Part model, mm, in its own coordinate system. A direction names the side the tool comes from. Coordinates: 2 decimals unless noted, no trailing zeros. Loops run counter-clockwise (first coordinate to the right, second up) from the corner with the lowest first, then second, coordinate; pieces in that order, holes last. Notation, with made-up numbers: M -31,-23.75 L 25,-23.75 A10 cw 25,-4.75 Z; hole C -5,20 d10. An arc over 180 degrees is marked long. Answer as CSV lines item,"result". Start each with the question number.
from build123d import *

# Parameters (mm, degrees)
F0_R     = 2.5
F1_DEPTH = 17
F2_T     = 0.4


# Not quite as in the source:
# - a shell that OpenCascade refuses in one call is made with other operations: the cavity is built on its own and cut out


with BuildPart() as f1:
    # F0 (on Front) → F1 (new body)
    with BuildSketch(Plane.XZ):
        with BuildLine():
            ThreePointArc((8.4418530872, -1.5193999292), (8.6686009191, 0.2448895048), (8.1079887938, 1.933038145))
            ThreePointArc((8.1079887938, 1.933038145), (-1.0644623598, 6.4400537212), (-9, 0))
            Line((-9, 0), (-14.990051355, -26.4365585686))
            ThreePointArc((-14.990051355, -26.4365585686), (-16.0266215588, -29.0388056628), (-17.8130271161, -31.1963326989))
            Line((-17.8130271161, -31.1963326989), (-31.2685862961, -43.0686485372))
            ThreePointArc((-31.2685862961, -43.0686485372), (-32.0681766379, -44.1518925803), (-32.3514207584, -45.4681505868))
            Line((-32.3514207584, -45.4681505868), (-32.3514207584, -45.4984797908))
            ThreePointArc((-32.3514207584, -45.4984797908), (-31.4935858742, -47.678906944), (-29.3800066519, -48.6903050507))
            Line((-29.3800066519, -48.6903050507), (-13.5882116102, -49.8212509157))
            ThreePointArc((-13.5882116102, -49.8212509157), (-12.2679323329, -50.4526148934), (-11.7310788719, -51.8140649305))
            Line((-11.7310788719, -51.8140649305), (-11.6569881297, -123.1658389017))
            Line((-11.6569881297, -123.1658389017), (0, -24.5))
            Line((0, -24.5), (8.4418530872, -1.5193999292))
        make_face()
        with Locations((0, -10)):
            Circle(F0_R, mode=Mode.SUBTRACT)
        Circle(F0_R, mode=Mode.SUBTRACT)
    extrude(amount=F1_DEPTH)

    # F2: shell of thickness 0.4, made by hand


with BuildPart() as f2_core1:
    # F2_t2: copy of F1
    add(f1.part)

    # the walls: a layer under each face that stays
    f2_faces = [f2_core1.faces().sort_by_distance(p)[0] for p in [
        (-16.0266215588, -8.5, -29.0388056628),
        (-24.5408067061, -8.5, -37.1324906181),
        (-32.0681766379, -8.5, -44.1518925803),
        (-32.3514207584, -8.5, -45.4833151888),
        (-31.4935858742, -8.5, -47.678906944),
        (-21.484109131, -8.5, -49.2557779832),
        (-12.2679323329, -8.5, -50.4526148934),
        (-11.6940335008, -8.5, -87.4899519161),
        (-2.5, -8.5, -10),
        (-2.5, -8.5, 0),
        (-11.8321233546, 0, -15.1109731503),
        (-11.8321233546, -17, -15.1109731503),
    ]]
    thicken(f2_faces, amount=-F2_T, mode=Mode.SUBTRACT)


with BuildPart() as f1_1:
    add(f1.part)

    # what is left inside the walls is the cavity
    f2_cavity = [f2_core1.part.solids().sort_by_distance(p)[0] for p in [
        (-5.634209, -11.2, -72.154379),
    ]]
    add(f2_cavity, mode=Mode.SUBTRACT)


solid = f1_1.part
Q1. Flat gauge pins, fed straight in: P1, Ø4, axis at x = -25.5, y = -3.5, coming from the -Z side; P2, Ø6, axis at x = -21, y = -12, coming from the +Z side; P3, Ø8, axis at x = -2, y = -7.5, coming from the +Z side. Where does each tip first touch, or does it go through?
Q2. Two-plate mould, pull along Z, no slides. Class faces 6 (the face through (-21.59, -8.38, -49.25)), 7 (the face through (-2.9, -8.4, 0.1)), 8 (the face through (-0.54, -8.38, -2.44)), 9 (the face through (-0.914, -0.197, 6.456)): +Z half, -Z half, draft (parallel to the pull), parting line (faces both ways), or undercut.
Q3. Slice it at A-A, the plane y = -3. State how many separate pieces and enclosed holes the cut face has, and give its area (3 significant figures).
Q4. Slice it at C-C, the plane z = -10. Write the cut outline in (x, y), and give its area (3 significant figures).
Q5. Tool access for faces 1 (the face through (-24.45, -8.38, -37.05)), 2 (the face through (-11.993, -8.387, -50.162)), 3 (the face through (4.16, -16.8, -13.17)), 4 (the face through (-31.697, -8.387, -44.301)), 5 (the face through (-2.9, -8.4, -9.9)): list every direction of +Z, -Z, +X, -X, +Y, -Y with a clear straight run to the whole face (end or side of a thin tool).
Q6. Wall check: L1, parallel to Z at x = 0, y = -4.5; L2, parallel to Y at x = -7, z = -64; L3, parallel to Z at x = 1, y = -13. Give the ranges that are in metal, low to high.
Q7. Slice it at B-B, the plane x = -4.5. Write the cut outline in (y, z).
Q8. Slice it at D-D, the plane x = -20. Write the cut outline in (y, z).
Solved:
1,P1,"stops at z = -49.11"
1,P2,"stops at z = -31.36"
1,P3,"stops at z = 2.9"
2,face 6,"-Z half"
2,face 7,"undercut"
2,face 8,"undercut"
2,face 9,"+Z half"
3,separate pieces,"3"
3,enclosed holes,"2"
3,area,"61.4 mm2"
4,outline,"M -11.27,-17 L -2.5,-17 L -2.5,0 L -11.27,0 L -11.27,-0.4 L -2.9,-0.4 L -2.9,-16.6 L -11.27,-16.6 Z; M 2.5,-17 L 5.33,-17 L 5.33,-16.6 L 2.9,-16.6 L 2.9,-0.4 L 5.33,-0.4 L 5.33,0 L 2.5,0 Z"
4,area,"22.2 mm2"
5,face 1,"+Z, -X, +Y, -Y"
5,face 2,"+Z, +X"
5,face 3,"-Z, +X, +Y, -Y"
5,face 4,"+X"
5,face 5,"none"
6,L1,"z = -12.9 to -12.5, -7.5 to -7.1, -2.9 to -2.5, 2.5 to 2.9"
6,L2,"y = -17 to -16.6, -0.4 to 0"
6,L3,"z = -12.72 to -12.29, -7.71 to -7.28, -2.72 to -2.29, 2.29 to 2.72"
7,outline,"M -17,-62.59 L -16.6,-62.59 L -16.6,5.36 L -17,5.36 Z; M -0.4,-62.59 L 0,-62.59 L 0,5.36 L -0.4,5.36 Z"
8,outline,"M -17,-49.36 L 0,-49.36 L 0,-33.13 L -17,-33.13 Z; hole M -16.6,-48.96 L -0.4,-48.96 L -0.4,-33.66 L -16.6,-33.66 Z"
